The listing builds one solid part. Answer for the finished solid, in the listing's coordinates (mm). Face numbers are marked on the shaded views. A direction names the side the tool comes from. Give positions to 0.01 mm unless a question says otherwise; leave off trailing zeros. Write each loop counter-clockwise with the first axis right and the second up, starting at its lowest first coordinate (ties: lowest second). Pieces come first, ordered by that corner, then holes. Notation, with made-up numbers: M 57.5,-29 L 65.5,-29 A12 ccw 65.5,-23 Z; hole C 57,59 d7. An arc over 180 degrees is marked long. Return JSON: item names as keys, results as strings.
from build123d import *

# Parameters (mm, degrees)
F0_W     = 17
F0_H     = 3
F0_W_2   = 57
F0_W_3   = 28.5
F0_H_2   = 19
F1_DEPTH = 100


# Not quite as in the source:
# - a feature of the source that left no trace in its solid (it failed there, or was rolled back) is left out


with BuildPart() as f1:
    # F0 (on Right) → F1 (new body)
    with BuildSketch(Plane.YZ):
        with Locations((-31.5, 1.5)):
            Rectangle(F0_W, F0_H)
        Polygon((-68.5, 22), (-40, 22), (-40, 25), (-71.5, 25), (-71.5, 0), (-40, 0), (-40, 3), (-68.5, 3), align=None)
        with Locations((-11.5, 23.5)):
            Rectangle(F0_W_2, F0_H)
        Polygon((17, 3), (17, 0), (48.5, 0), (48.5, 25), (17, 25), (17, 22), (45.5, 22), (45.5, 3), align=None)
        with Locations((8.5, 1.5)):
            Rectangle(F0_W, F0_H)
        with Locations((31.25, 12.5)):
            Rectangle(F0_W_3, F0_H_2)
        with Locations((-54.25, 12.5)):
            Rectangle(F0_W_3, F0_H_2)
    extrude(amount=F1_DEPTH)


solid = f1.part
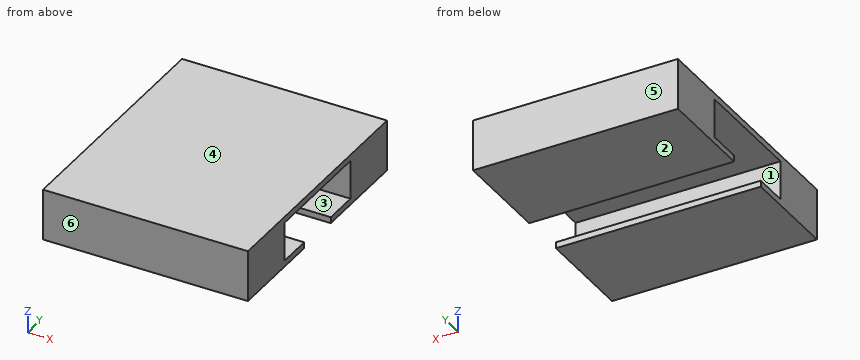
Item 1: Determine the mould class of the marked faces 3, 4, 5 and 6 for opening direction Y: +Y half, -Y half, draft (parallel to the pull), parting line (faces both ways), or undercut.
Geometry results:
{"face 3": "undercut", "face 4": "draft", "face 5": "+Y half", "face 6": "-Y half"}
Item 2: A cutting plane is placed at D-D, the plane y = -6.5. Write down the section's boundary in (x, z).
Geometry results:
{"outline": "M 0,22 L 100,22 L 100,25 L 0,25 Z"}
Item 3: A cutting plane is placed at A-A, the plane y = -27.5. Write down the section's boundary in (x, z).
Geometry results:
{"outline": "M 0,0 L 100,0 L 100,3 L 0,3 Z; M 0,22 L 100,22 L 100,25 L 0,25 Z"}
Item 4: A cutting plane is placed at C-C, the plane z = 4.75. Write down the section's boundary in (x, y).
Geometry results:
{"outline": "M 0,-71.5 L 100,-71.5 L 100,-40 L 0,-40 Z; M 0,17 L 100,17 L 100,48.5 L 0,48.5 Z"}
Item 5: A cutting plane is placed at B-B, the plane x = 61. Write down the section's boundary in (y, z), plus the area to 3 significant figures.
Geometry results:
{"outline": "M -71.5,0 L -23,0 L -23,3 L -40,3 L -40,22 L 17,22 L 17,3 L 0,3 L 0,0 L 48.5,0 L 48.5,25 L -71.5,25 Z", "area": "1,850 mm2"}
Item 6: Which of the six approach directions +Z, -Z, +X, -X, +Y, -Y give full straight-line access (tool end or side, diameter ignored) to the marked faces 1 and 2?
Geometry results:
{"face 1": "+X, -X", "face 2": "-Z, +X, -X, +Y, -Y"}
Item 7: Find the intervals of material crossed by line 1 (Y direction, x = 79, z = 9); line 2 (Z direction, x = 87, y = 8); line 3 (Y direction, x = 37.5, z = 2.25), in increasing order.
Geometry results:
{"line 1": "y = -71.5 to -40, 17 to 48.5", "line 2": "z = 0 to 3, 22 to 25", "line 3": "y = -71.5 to -23, 0 to 48.5"}
